```python
from build123d import *

# Parameters (mm, degrees)
F1_DEPTH = 29
F3_DEPTH = 28
F4_W     = 6
F4_H     = 7
F5_DEPTH = 44.45


# Not quite as in the source:
# - a feature names something its author has since deleted; it is built from what else it names


with BuildPart() as f1:
    # F0 (on Top) → F1 (new body)
    with BuildSketch(Plane.XY):
        with BuildLine():
            Line((-33.65, -25), (40, -25))
            Line((40, -25), (40, 18.65))
            ThreePointArc((40, 18.65), (38.1401280605, 23.1401280605), (33.65, 25))
            Line((33.65, 25), (-40, 25))
            Line((-40, 25), (-40, -18.65))
            ThreePointArc((-40, -18.65), (-38.1401280605, -23.1401280605), (-33.65, -25))
        make_face()
    extrude(amount=F1_DEPTH)

    # F2 (on face) → F3 (cut)
    with BuildSketch(Plane.XY.offset(29)):
        with BuildLine():
            Line((33.666, 24), (-39, 24))
            Line((-39, 24), (-39, -18.666))
            ThreePointArc((-39, -18.666), (-37.4377075708, -22.4377075708), (-33.666, -24))
            Line((-33.666, -24), (39, -24))
            Line((39, -24), (39, 18.666))
            ThreePointArc((39, 18.666), (37.4377075708, 22.4377075708), (33.666, 24))
        make_face()
    extrude(amount=-F3_DEPTH, mode=Mode.SUBTRACT)

    # F4 (on face) → F5 (cut)
    with BuildSketch(Plane.YZ.offset(-39)):
        with Locations((6, 25.5)):
            Rectangle(F4_W, F4_H)
    extrude(amount=-F5_DEPTH, mode=Mode.SUBTRACT)


solid = f1.part
```
Can you work these out from the model? Positions are in its coordinate system, mm. A direction names the side the tool comes from. Coordinates: 2 decimals unless noted, no trailing zeros. Loops run counter-clockwise (first coordinate to the right, second up) from the corner with the lowest first, then second, coordinate; pieces in that order, holes last. Notation, with made-up numbers: (69, 75.5) - (83, 75.5) arc R17 cw to (83, 81.5) - close; hole circle Ø10 at (54.25, 21). An arc over 180 degrees is marked (long way). Use a Markdown table: item, result.
Item 1: If I drill on probe 1 along X at (y, z) = (-12, 6); probe 2 along Y at (x, z) = (3.5, 23); probe 3 along Z at (x, y) = (22, -13), over which ranges is the centre line in solid material (lowest first)? Write a range as from..to.
Numbers:
| item | result |
|---|---|
| probe 1 | x = -40..-39, 39..40 |
| probe 2 | y = -25..-24, 24..25 |
| probe 3 | z = 0..1 |
Item 2: Will these pins go through, and if not, where does the flat tip stop? pin 1 (12 mm diameter, centred on x = 18.5, y = -11, fed in from +Z); pin 2 (0.5 mm diameter, centred on x = -39.5, y = 7, fed in from +Z); pin 3 (1.1 mm diameter, centred on x = -39.5, z = 27, fed in from -Y).
Numbers:
| item | result |
|---|---|
| pin 1 | stops at z = 1 |
| pin 2 | stops at z = 22 |
| pin 3 | stops at y = -22.15 |
Item 3: We'd pull the mould along Y, two halves only. Please class faces 1 (the face through (-37.479, -22.396, 15.196)), 2 (the face through (-3.1, 24.2, 29)), 3 (the face through (-38.19, -23.09, 14.3)): released by +Y, released by -Y, zero draft, split by the parting line, or undercut.
Numbers:
| item | result |
|---|---|
| face 1 | undercut |
| face 2 | zero draft |
| face 3 | released by -Y |
Item 4: I want a section at B-B on y = 0.5. Please give me the cut outline in (x, z), and give its area (3 significant figures).
Numbers:
| item | result |
|---|---|
| outline | (-40, 0) - (40, 0) - (40, 29) - (39, 29) - (39, 1) - (-39, 1) - (-39, 29) - (-40, 29) - close |
| area | 136 mm2 |
Item 5: For faces 4 (the face through (-39, 3, 15)), 5 (the face through (40, -3, 14)), which set-ups out of +Z, -Z, +X, -X, +Y, -Y let a thin tool reach every point of the face, with its end or its side?
Numbers:
| item | result |
|---|---|
| face 4 | +Z |
| face 5 | +Z, -Z, +X, +Y, -Y |
Item 6: I want a section at C-C on x = 30.5. Please give me the cut outline in (y, z), and give its area (3 significant figures).
Numbers:
| item | result |
|---|---|
| outline | (-25, 0) - (25, 0) - (25, 29) - (24, 29) - (24, 1) - (-24, 1) - (-24, 29) - (-25, 29) - close |
| area | 106 mm2 |
Item 7: I want a section at A-A on z = 16.25. Please give me the cut outline in (x, y), and give its area (3 significant figures).
Numbers:
| item | result |
|---|---|
| outline | (-40, -18.65) arc R6.35 ccw to (-33.65, -25) - (40, -25) - (40, 18.65) arc R6.35 ccw to (33.65, 25) - (-40, 25) - close; hole (-39, -18.67) arc R5.33 ccw to (-33.67, -24) - (39, -24) - (39, 18.67) arc R5.33 ccw to (33.67, 24) - (-39, 24) - close |
| area | 251 mm2 |
Item 8: I want a section at D-D on z = 23. Please give me the cut outline in (x, y), and give its area (3 significant figures).
Numbers:
| item | result |
|---|---|
| outline | (-40, -18.65) arc R6.35 ccw to (-33.65, -25) - (40, -25) - (40, 18.65) arc R6.35 ccw to (33.65, 25) - (-40, 25) - (-40, 9) - (-39, 9) - (-39, 24) - (33.67, 24) arc R5.33 cw to (39, 18.67) - (39, -24) - (-33.67, -24) arc R5.33 cw to (-39, -18.67) - (-39, 3) - (-40, 3) - close |
| area | 245 mm2 |
